The listing builds one solid part. Answer for the finished solid, in the listing's coordinates (mm). Coordinates: 2 decimals unless noted, no trailing zeros. Order: outer loops, then holes, each group sorted by start corner. A loop starts at its lowest first (then second) coordinate and runs counter-clockwise, first axis right, second up. Notation, with made-up numbers: (31, 18) -> (65, 18) arc R29 cw to (65, 55) -> close; hole circle Ø5 at (-23, 61). An arc over 180 degrees is marked (long way). One line per question, with ' | ' between items.
from build123d import *

# Parameters (mm, degrees)
CROQUIS1_W              = 202
CROQUIS1_H              = 188
SALIENTE_EXTRUIR1_DEPTH = 12.7
CROQUIS2_R              = 2
CROQUIS2_R_2            = 4.765
CORTAR_EXTRUIR1_DEPTH   = 12.7


with BuildPart() as part:
    # Croquis1 → Saliente-Extruir1 (new body)
    with BuildSketch(Plane.XY):
        Rectangle(CROQUIS1_W, CROQUIS1_H)
    extrude(amount=SALIENTE_EXTRUIR1_DEPTH)

    # Croquis2 → Cortar-Extruir1 (cut)
    with BuildSketch(Plane.XY.offset(12.7)):
        with Locations((-74, -76)):
            Circle(CROQUIS2_R)
        with Locations((-49, -76)):
            Circle(CROQUIS2_R)
        with Locations((-24, -76)):
            Circle(CROQUIS2_R)
        with Locations((1, -76)):
            Circle(CROQUIS2_R)
        with Locations((26, -76)):
            Circle(CROQUIS2_R)
        with Locations((51, -76)):
            Circle(CROQUIS2_R)
        with Locations((76, -76)):
            Circle(CROQUIS2_R)
        with Locations((-49, -51)):
            Circle(CROQUIS2_R)
        with Locations((-24, -51)):
            Circle(CROQUIS2_R)
        with Locations((1, -51)):
            Circle(CROQUIS2_R)
        with Locations((26, -51)):
            Circle(CROQUIS2_R)
        with Locations((51, -51)):
            Circle(CROQUIS2_R)
        with Locations((76, -51)):
            Circle(CROQUIS2_R)
        with Locations((-49, -26)):
            Circle(CROQUIS2_R)
        with Locations((-24, -26)):
            Circle(CROQUIS2_R)
        with Locations((1, -26)):
            Circle(CROQUIS2_R)
        with Locations((26, -26)):
            Circle(CROQUIS2_R)
        with Locations((51, -26)):
            Circle(CROQUIS2_R)
        with Locations((76, -26)):
            Circle(CROQUIS2_R)
        with Locations((-49, -1)):
            Circle(CROQUIS2_R)
        with Locations((-24, -1)):
            Circle(CROQUIS2_R)
        with Locations((1, -1)):
            Circle(CROQUIS2_R)
        with Locations((26, -1)):
            Circle(CROQUIS2_R)
        with Locations((51, -1)):
            Circle(CROQUIS2_R)
        with Locations((76, -1)):
            Circle(CROQUIS2_R)
        with Locations((-49, 24)):
            Circle(CROQUIS2_R)
        with Locations((-24, 24)):
            Circle(CROQUIS2_R)
        with Locations((1, 24)):
            Circle(CROQUIS2_R)
        with Locations((26, 24)):
            Circle(CROQUIS2_R)
        with Locations((51, 24)):
            Circle(CROQUIS2_R)
        with Locations((76, 24)):
            Circle(CROQUIS2_R)
        with Locations((-49, 49)):
            Circle(CROQUIS2_R)
        with Locations((-24, 49)):
            Circle(CROQUIS2_R)
        with Locations((1, 49)):
            Circle(CROQUIS2_R)
        with Locations((26, 49)):
            Circle(CROQUIS2_R)
        with Locations((51, 49)):
            Circle(CROQUIS2_R)
        with Locations((76, 49)):
            Circle(CROQUIS2_R)
        with Locations((-49, 74)):
            Circle(CROQUIS2_R)
        with Locations((-24, 74)):
            Circle(CROQUIS2_R)
        with Locations((1, 74)):
            Circle(CROQUIS2_R)
        with Locations((26, 74)):
            Circle(CROQUIS2_R)
        with Locations((51, 74)):
            Circle(CROQUIS2_R)
        with Locations((76, 74)):
            Circle(CROQUIS2_R)
        with Locations((-74, -51)):
            Circle(CROQUIS2_R)
        with Locations((-74, -26)):
            Circle(CROQUIS2_R)
        with Locations((-74, -1)):
            Circle(CROQUIS2_R)
        with Locations((-74, 24)):
            Circle(CROQUIS2_R)
        with Locations((-74, 49)):
            Circle(CROQUIS2_R)
        with Locations((-74, 74)):
            Circle(CROQUIS2_R)
        with Locations((39, -61)):
            Circle(CROQUIS2_R_2)
        with Locations((-62.6, 40.6)):
            Circle(CROQUIS2_R_2)
    extrude(amount=-CORTAR_EXTRUIR1_DEPTH, mode=Mode.SUBTRACT)


solid = part.part
Item 1: Find the intervals of material crossed by L1, parallel to Y at x = 35, z = 11.5; L2, parallel to X at y = 39.5, z = 11.25, in increasing order.
Computed values:
L1: y = -94 to -63.59, -58.41 to 94 | L2: x = -101 to -67.24, -57.96 to 101
Item 2: Section C-C, the plane z = 2.5 is taken. Count the separate pieces of the cut face and the enclosed holes in it, plus the area to 3 significant figures.
Computed values:
separate pieces: 1 | enclosed holes: 51 | area: 37,200 mm^2
Item 3: Section A-A, the plane y = -61 is taken. Give the vertices of the cut face in (x, z) (3 decimals).
Computed values:
outline: (-101, 0) -> (34.235, 0) -> (34.235, 12.7) -> (-101, 12.7) -> close; (43.765, 0) -> (101, 0) -> (101, 12.7) -> (43.765, 12.7) -> close
Item 4: Section B-B, the plane x = 39 is taken. Give the vertices of the cut face in (y, z) (3 decimals), plus the area to 3 significant figures.
Computed values:
outline: (-94, 0) -> (-65.765, 0) -> (-65.765, 12.7) -> (-94, 12.7) -> close; (-56.235, 0) -> (94, 0) -> (94, 12.7) -> (-56.235, 12.7) -> close | area: 2,270 mm^2
Item 5: Determine the mould class of faces 1 (the face through (41.56, -56.98, 6.44)), 2 (the face through (-1, -94, 6)), 3 (the face through (101, -1, 6)) for opening direction Y: pulls with the +Y half, pulls with the -Y half, needs draft (parallel to the pull), parting line crosses it, or undercut.
Computed values:
face 1: undercut | face 2: pulls with the -Y half | face 3: needs draft
Item 6: This flat-tipped pin is pushed along its axis until it touches: pin 1 Ø3 at (x, y) = (-24, 74) entering from +Z. Where does it stop, or does it pass through?
Computed values:
pin 1: passes through
